Design review of the part built by this model. Coordinates are the model's own, in mm. A direction names the side the tool comes from. Give positions to 0.01 mm unless a question says otherwise; leave off trailing zeros. Loops run counter-clockwise (first coordinate to the right, second up) from the corner with the lowest first, then second, coordinate; pieces in that order, holes last. Notation, with made-up numbers: (29, -4) -> (34, -4) arc R23 cw to (34, 6) -> close; hole circle Ø1 at (8, -7). An arc over 180 degrees is marked (long way). Answer in a Markdown table with one row per item. Add a question column.
(1) Consider section B-B on z = 19.5. Write out the cut boundary in (x, y) (3 decimals).
(2) Draft analysis for pull direction X (two halves, no side actions). For faces 1 (the flat face through (-11, 6, 7)), 2 (the cylindrical face through (-8.27, 3.04, -12.38)), 3 (the flat face through (-56, 3, 0)), state which applies: +X half, -X half, draft (parallel to the pull), parting line (faces both ways), or undercut.
(3) Consider section C-C on y = 1.45. Count the separate pieces of the cut face and the enclosed holes in it, then the cut area to 3 significant figures.
(4) Consider section A-A on x = 0. Write out the cut boundary in (y, z).
(5) Consider section D-D on z = 10. Write out the cut boundary in (x, y), then the cut area to 3 significant figures.
(6) For pin 1 (21.5 mm diameter, centred on x = 0, z = 0, fed in from -Y); pin 2 (1.5 mm diameter, centred on x = -43.5, y = 4, fed in from +Z); pin 3 (1.5 mm diameter, centred on y = 4, z = -1, fed in from +X); pin 4 (1.5 mm diameter, centred on x = -9.5, y = 3, fed in from +Z), all flat-tipped, find the tip position at first contact; note any pin that passes through.
(7) For faces 4 (the flat face through (-21.3, 3, 0)), 5 (the flat face through (-28.636, 2.958, 31.667)), list the 3-axis set-ups (+Z, -Z, +X, -X, +Y, -Y) from which the entire face can be reached by the end or side of a thin tool; tool diameter is ignored.
(8) For line 1 (Z direction, x = -8.5, y = 4.3); line 2 (Z direction, x = -2.5, y = 0.6); line 3 (X direction, y = 3.3, z = 10), list the stretches that pass through material, from the lowest coordinate up.
from build123d import *

# Parameters (mm, degrees)
EXTRUDE_1_DEPTH     = 6
SKETCH_4_R          = 12
CUT_EXTRUDE_2_DEPTH = 6
SKETCH_5_R          = 1.6
CUT_EXTRUDE_3_DEPTH = 6
SKETCH_6_R          = 4.5
SKETCH_6_R_2        = 2.1
CUT_EXTRUDE_4_DEPTH = 6
SKETCH_7_W          = 5.6
SKETCH_7_H          = 7
CUT_EXTRUDE_5_DEPTH = 6
FILLET_2_R          = 1


with BuildPart() as part:
    # 草图1 → 凸台-拉伸1 (new body)
    with BuildSketch(Plane(origin=(0, 0, 0), x_dir=(1, 0, 0), z_dir=(0, 1, 0))):
        with BuildLine():
            Line((-56, -30), (-56, 30))
            Line((-56, 30), (-2.028111517, 33.288275168))
            ThreePointArc((-2.028111517, 33.288275168), (33.35, 0), (-2.028111517, -33.288275168))
            Line((-2.028111517, -33.288275168), (-56, -30))
        make_face()
    extrude(amount=EXTRUDE_1_DEPTH)

    # 草图4 → 切除-拉伸2 (cut)
    with BuildSketch(Plane(origin=(0, 6, 0), x_dir=(1, 0, 0), z_dir=(0, 1, 0))):
        with Locations(Location((0, 0, 0), (0, 0, 270))):
            Circle(SKETCH_4_R)
    extrude(amount=-CUT_EXTRUDE_2_DEPTH, mode=Mode.SUBTRACT)

    # 草图5 → 切除-拉伸3 (cut)
    with BuildSketch(Plane(origin=(0, 6, 0), x_dir=(1, 0, 0), z_dir=(0, 1, 0))):
        with Locations(Location((-46, 20, 0), (0, 0, 270))):
            Circle(SKETCH_5_R)
        with Locations(Location((-46, 10, 0), (0, 0, 270))):
            Circle(SKETCH_5_R)
        with Locations(Location((-46, -20, 0), (0, 0, 90))):
            Circle(SKETCH_5_R)
        with Locations(Location((-46, -10, 0), (0, 0, 90))):
            Circle(SKETCH_5_R)
    extrude(amount=-CUT_EXTRUDE_3_DEPTH, mode=Mode.SUBTRACT)

    # 草图6 → 切除-拉伸4 (cut)
    with BuildSketch(Plane(origin=(0, 6, 0), x_dir=(1, 0, 0), z_dir=(0, 1, 0))):
        with Locations(Location((-9.625, 16.670989023, 0), (0, 0, 270))):
            Circle(SKETCH_6_R)
        with Locations(Location((29, 0, 0), (0, 0, 270))):
            Circle(SKETCH_6_R_2)
        with Locations(Location((-14.5, -25.11473671, 0), (0, 0, 270))):
            Circle(SKETCH_6_R_2)
        with Locations(Location((-14.5, 25.11473671, 0), (0, 0, 270))):
            Circle(SKETCH_6_R_2)
    extrude(amount=-CUT_EXTRUDE_4_DEPTH, mode=Mode.SUBTRACT)

    # 草图7 → 切除-拉伸5 (cut)
    with BuildSketch(Plane(origin=(0, 6, 0), x_dir=(1, 0, 0), z_dir=(0, 1, 0))):
        with Locations((-18.5, 0)):
            Rectangle(SKETCH_7_W, SKETCH_7_H)
    extrude(amount=-CUT_EXTRUDE_5_DEPTH, mode=Mode.SUBTRACT)

    # 圆角2
    fillet_2_edges = [part.edges().sort_by_distance(p)[0] for p in [
        (-15.7, 3, 3.5),
        (-15.7, 3, -3.5),
        (-21.3, 3, -3.5),
        (-21.3, 3, 3.5),
    ]]
    fillet(fillet_2_edges, radius=FILLET_2_R)


solid = part.part
Values follow:
| question | item | result |
|---|---|---|
| 1 | outline | (-56, 0) -> (-47.52, 0) -> (-47.52, 6) -> (-56, 6) -> close; (-44.48, 0) -> (27.055, 0) -> (27.055, 6) -> (-44.48, 6) -> close |
| 2 | face 1 | draft |
| 2 | face 2 | undercut |
| 2 | face 3 | -X half |
| 3 | separate pieces | 1 |
| 3 | enclosed holes | 10 |
| 3 | area | 4,670 mm2 |
| 4 | outline | (0, -33.35) -> (6, -33.35) -> (6, -12) -> (0, -12) -> close; (0, 12) -> (6, 12) -> (6, 33.35) -> (0, 33.35) -> close |
| 5 | outline | (-56, 0) -> (-47.6, 0) -> (-47.6, 6) -> (-56, 6) -> close; (-44.4, 0) -> (-6.63, 0) -> (-6.63, 6) -> (-44.4, 6) -> close; (6.63, 0) -> (31.82, 0) -> (31.82, 6) -> (6.63, 6) -> close |
| 5 | area | 428 mm2 |
| 6 | pin 1 | through |
| 6 | pin 2 | z = 30.81 |
| 6 | pin 3 | x = 33.35 |
| 6 | pin 4 | z = 32.88 |
| 7 | face 4 | +Y, -Y |
| 7 | face 5 | +Z, -X, +Y, -Y |
| 8 | line 1 | -32.89 to -21.03, -12.31 to -8.47, 8.47 to 32.89 |
| 8 | line 2 | -33.26 to -11.74, 11.74 to 33.26 |
| 8 | line 3 | -56 to -47.6, -44.4 to -6.63, 6.63 to 31.82 |
